```python
from build123d import *

# Parameters (mm, degrees)
F0_W     = 27.5
F0_H     = 66
F1_DEPTH = 30
F2_W     = 66
F2_H     = 30
F3_DEPTH = 0.5
F4_W     = 28.5
F4_H     = 66
F5_DEPTH = 0.5
F7_DEPTH = 0.5
F8_W     = 20.5
F8_H     = 58
F9_DEPTH = 28.5
F10_R    = 10.24999


# Not quite as in the source:
# - two fillets or chamfers of one size are made in one step
# - a fillet or chamfer is up to 0.001 mm smaller than in the source, because OpenCascade refuses the exact size
# - a pattern or mirror of a feature is missing from the dataset's text; its kind, count and spacing are read off the source's solid


with BuildPart() as f1:
    # F0 (on Top) → F1 (new body)
    with BuildSketch(Plane.XY):
        Rectangle(F0_W, F0_H)
    extrude(amount=F1_DEPTH)

    # F2 (on face) → F3 (join)
    with BuildSketch(Plane.YZ.offset(13.75)):
        with Locations((0, 15)):
            Rectangle(F2_W, F2_H)
        Polygon((28.3744677029, 1.8), (-29.8744677029, 1.8), (-0.75, 14.0239419294), align=None, mode=Mode.SUBTRACT)
        Polygon((-31.2, 3.7331419218), (-31.2, 26.8042280979), (-3.0755322971, 15), align=None, mode=Mode.SUBTRACT)
        Polygon((-0.0901844103, 16.195951202), (-28.3744677029, 28.2), (29.8744677029, 28.2), align=None, mode=Mode.SUBTRACT)
        Polygon((31.2, 27.4337988451), (31.2, 2.9161768244), (2.1548442575, 15.2431452425), align=None, mode=Mode.SUBTRACT)
    f3 = extrude(amount=F3_DEPTH)

    # F3_copies: F3 across plane
    add(f3.mirror(Plane(origin=(0, 0, 0), x_dir=(0, 0, -1), z_dir=(-1, 0, 0))))

    # F4 (on face) → F5 (join)
    with BuildSketch(Plane.XY.offset(30)):
        Rectangle(F4_W, F4_H)
        Polygon((0.25, -2.338037696), (12.2876657229, -31.2), (-11.3137418755, -31.2), align=None, mode=Mode.SUBTRACT)
        Polygon((-0.7251421589, 0), (-12.45, -28.111962304), (-12.45, 28.111962304), align=None, mode=Mode.SUBTRACT)
        Polygon((1.1867507353, 0), (12.45, 28.111962304), (12.45, -28.111962304), align=None, mode=Mode.SUBTRACT)
        Polygon((0.25, 2.338037696), (-11.3137418755, 31.2), (12.2876657229, 31.2), align=None, mode=Mode.SUBTRACT)
    extrude(amount=F5_DEPTH)

    # F6 (on face) → F7 (cut)
    with BuildSketch(Plane.XZ.offset(33)):
        Polygon((0, 14.0644738981), (-10.9635152767, 2.3), (10.9635152767, 2.3), align=None)
        Polygon((-1.1048121354, 15.25), (-11.95, 26.8875018716), (-11.95, 3.6124981284), align=None)
        Polygon((0, 16.4355261019), (10.9635152767, 28.2), (-10.9635152767, 28.2), align=None)
        Polygon((1.1048121354, 15.25), (11.95, 3.6124981284), (11.95, 26.8875018716), align=None)
    f7 = extrude(amount=-F7_DEPTH, mode=Mode.SUBTRACT)

    # F7_copies: F7 across plane
    add(f7.mirror(Plane.ZX), mode=Mode.SUBTRACT)

    # F8 (on face) → F9 (cut)
    with BuildSketch(Plane(origin=(0, 0, 0), x_dir=(1, 0, 0), z_dir=(0, 0, -1))):
        Rectangle(F8_W, F8_H)
    extrude(amount=-F9_DEPTH, mode=Mode.SUBTRACT)

    # F10 (radius 10.25 in the source; OpenCascade refuses exactly that, so slightly less here)
    f10_edges = [f1.edges().sort_by_distance(p)[0] for p in [
        (-10.25, 0, 28.5),
        (10.25, 0, 28.5),
    ]]
    fillet(f10_edges, radius=F10_R)


solid = f1.part
```
Input: part model. Units: mm. Frame: model coordinates. A direction names the side the tool comes from. Coordinates: 2 decimals unless noted, no trailing zeros. Answer in a Markdown table with one row per item.
1. First-contact query: pin 1 (6 mm diameter, centred on y = 16, z = 13, fed in from -X); pin 2 (3.5 mm diameter, centred on x = -1, z = 23, fed in from -Y); pin 3 (1 mm diameter, centred on y = 2, z = 11.5, fed in from +X). Flat tips, straight axial feed; report the tip coordinate or a pass-through.
Response:
| item | result |
|---|---|
| pin 1 | stops at x = -13.75 |
| pin 2 | stops at y = -32.5 |
| pin 3 | stops at x = 13.75 |
2. Draft query along Z for faces 1 (the flat face through (-5.613, -16.971, 30.246)), 2 (the flat face through (13.75, 0, 23)), 3 (the flat face through (8, 0, 30)). Return one class per face: pulls with the +Z half, pulls with the -Z half, needs draft (parallel to the pull), parting line crosses it, or undercut.
Response:
| item | result |
|---|---|
| face 1 | needs draft |
| face 2 | undercut |
| face 3 | pulls with the +Z half |
3. Material intervals for line 1 (X direction, y = 16.5, z = 7); line 2 (Y direction, x = -8, z = 2), sorted ascending.
Response:
| item | result |
|---|---|
| line 1 | x = -14.25 to -10.25, 10.25 to 14.25 |
| line 2 | y = -33 to -29, 29 to 33 |
4. Reachability of faces 4 (the flat face through (-13.996, -16.941, 9.445)), 5 (the flat face through (0, 32.5, 24)), 6 (the flat face through (1, -20, 30)) from +Z, -Z, +X, -X, +Y, -Y: full face, straight path, thin tool, end or side. Return the list, or none.
Response:
| item | result |
|---|---|
| face 4 | -X |
| face 5 | +Y |
| face 6 | +Z |
